```python
from build123d import *

# Parameters (mm, degrees)
SKETCH1_W           = 37.85108
SKETCH1_H           = 25.4
SKETCH1_R           = 8.309045905
BOSS_EXTRUDE1_DEPTH = 1.41224


with BuildPart() as part:
    # Sketch1 → Boss-Extrude1 (new body)
    with BuildSketch(Plane.XY):
        with Locations((18.92554, -12.7)):
            Rectangle(SKETCH1_W, SKETCH1_H)
        with Locations((9.46277, -12.7)):
            Circle(SKETCH1_R, mode=Mode.SUBTRACT)
        with Locations(Location((28.38831, -12.7, 0), (0, 0, 180))):
            Circle(SKETCH1_R, mode=Mode.SUBTRACT)
    extrude(amount=-BOSS_EXTRUDE1_DEPTH)


solid = part.part
```
Could you check a few things on this model? Use its own coordinates, in mm. Coordinates: 2 decimals unless noted, no trailing zeros. Order: outer loops, then holes, each group sorted by start corner. A loop starts at its lowest first (then second) coordinate and runs counter-clockwise, first axis right, second up. Notation, with made-up numbers: M 70.5,10 L 117.5,10 A16 cw 117.5,36 Z; hole C 41.5,6 d3. An arc over 180 degrees is marked long. Use one line per item in the form item = value. Start each with the question number.
1. Please list where these lines run through material, in increasing order: line 1 (X direction, y = -18.5, z = -0.65); line 2 (Y direction, x = 32.5, z = -0.4); line 3 (Y direction, x = 33, z = -1.2).
2. For pin 1 (5 mm diameter, centred on x = 21, y = -13, fed in from +Z); pin 2 (13.5 mm diameter, centred on x = 9.46, y = -12.7, fed in from +Z), each with a flat end and sliding along its axis, tell me the tip position at first contact or that it passes through.
3. Suppose I cut it at D-D on y = -5.75. Write out the boundary of the cut face in (x, z), then the cut area to 3 significant figures.
4. We'd pull the mould along X, two halves only. Please class faces 1 (the cylindrical face through (3.34, -7.08, -0.7)), 2 (the flat face through (0, -13, -1)), 3 (the flat face through (19, 0, -1)): +X half, -X half, draft (parallel to the pull), parting line (faces both ways), or undercut.
5. Suppose I cut it at A-A on y = -12.7. Write out the boundary of the cut face in (x, z), then the cut area to 3 significant figures.
6. Suppose I cut it at C-C on x = 5.5. Write out the boundary of the cut face in (y, z), then the cut area to 3 significant figures.
7. Suppose I cut it at B-B on z = -0.5. Write out the boundary of the cut face in (x, y), then the cut area to 3 significant figures.
Geometry says:
q1.line_1 = 0 to 3.51, 15.41 to 22.44, 34.34 to 37.85
q1.line_2 = -25.4 to -19.92, -5.48 to 0
q1.line_3 = -25.4 to -19.61, -5.79 to 0
q2.pin_1 = 0
q2.pin_2 = through
q3.outline = M 0,-1.41 L 4.91,-1.41 L 4.91,0 L 0,0 Z; M 14.02,-1.41 L 23.83,-1.41 L 23.83,0 L 14.02,0 Z; M 32.94,-1.41 L 37.85,-1.41 L 37.85,0 L 32.94,0 Z
q3.area = 27.7 mm^2
q4.face_1 = undercut
q4.face_2 = -X half
q4.face_3 = draft
q5.outline = M 0,-1.41 L 1.15,-1.41 L 1.15,0 L 0,0 Z; M 17.77,-1.41 L 20.08,-1.41 L 20.08,0 L 17.77,0 Z; M 36.7,-1.41 L 37.85,-1.41 L 37.85,0 L 36.7,0 Z
q5.area = 6.52 mm^2
q6.outline = M -25.4,-1.41 L -20,-1.41 L -20,0 L -25.4,0 Z; M -5.4,-1.41 L 0,-1.41 L 0,0 L -5.4,0 Z
q6.area = 15.2 mm^2
q7.outline = M 0,-25.4 L 37.85,-25.4 L 37.85,0 L 0,0 Z; hole C 9.46,-12.7 d16.62; hole C 28.39,-12.7 d16.62
q7.area = 528 mm^2
